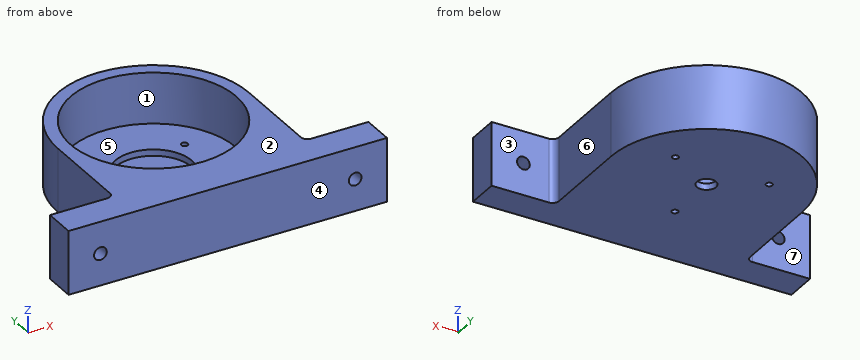
```python
from build123d import *

# Parameters (mm, degrees)
PAD_DEPTH       = 10
SKETCH001_R     = 13
POCKET_DEPTH    = 8
SKETCH002_R     = 6
POCKET001_DEPTH = 1
SKETCH003_R     = 1.5
POCKET002_DEPTH = 1
SKETCH004_R     = 0.5
POCKET003_DEPTH = 2
SKETCH005_R     = 1
POCKET004_DEPTH = 5
FILLET_R        = 1
FILLET001_R     = 1


with BuildPart() as part:
    # Sketch → Pad (new body)
    with BuildSketch(Plane.XY):
        with BuildLine():
            ThreePointArc((15, 0), (0, 15), (-15, 0))
            Line((-15, 0), (-15, -15))
            Line((-15, -15), (-25, -15))
            Line((-25, -15), (-25, -20))
            Line((-25, -20), (25, -20))
            Line((25, -15), (25, -20))
            Line((15, -15), (25, -15))
            Line((15, 0), (15, -15))
        make_face()
    extrude(amount=PAD_DEPTH)

    # Sketch001 (on Face10 of Pad) → Pocket (cut)
    with BuildSketch(Plane.XY.offset(10)):
        Circle(SKETCH001_R)
    extrude(amount=-POCKET_DEPTH, mode=Mode.SUBTRACT)

    # Sketch002 (on Face12 of Pocket) → Pocket001 (cut)
    with BuildSketch(Plane.XY.offset(2)):
        Circle(SKETCH002_R)
    extrude(amount=-POCKET001_DEPTH, mode=Mode.SUBTRACT)

    # Sketch003 (on Face14 of Pocket001) → Pocket002 (cut)
    with BuildSketch(Plane.XY.offset(1)):
        Circle(SKETCH003_R)
    extrude(amount=-POCKET002_DEPTH, mode=Mode.SUBTRACT)

    # Sketch004 (on Face14 of Pocket002) → Pocket003 (cut)
    with BuildSketch(Plane.XY.offset(2)):
        with Locations((0, -8.5)):
            Circle(SKETCH004_R)
        with Locations((7.361216, 4.25)):
            Circle(SKETCH004_R)
        with Locations((-7.361216, 4.25)):
            Circle(SKETCH004_R)
    extrude(amount=-POCKET003_DEPTH, mode=Mode.SUBTRACT)

    # Sketch005 (on Face6 of Pocket003) → Pocket004 (cut)
    with BuildSketch(Plane(origin=(0, -15, 0), x_dir=(-1, 0, 0), z_dir=(0, 1, 0))):
        with Locations((-20, 5)):
            Circle(SKETCH005_R)
        with Locations((20, 5)):
            Circle(SKETCH005_R)
    extrude(amount=-POCKET004_DEPTH, mode=Mode.SUBTRACT)

    # Fillet
    fillet_edges = [part.edges().sort_by_distance(p)[0] for p in [
        (-15, -15, 5),
    ]]
    fillet(fillet_edges, radius=FILLET_R)

    # Fillet001
    fillet001_edges = [part.edges().sort_by_distance(p)[0] for p in [
        (15, -15, 5),
    ]]
    fillet(fillet001_edges, radius=FILLET001_R)


solid = part.part
```
The model under review builds one solid part; all positions refer to its coordinate system, in mm. Face numbers are marked on the shaded views. A direction names the side the tool comes from. Round coordinates to 2 decimals unless told otherwise and drop trailing zeros. Loops run counter-clockwise (first coordinate to the right, second up) from the corner with the lowest first, then second, coordinate; pieces in that order, holes last. Notation, with made-up numbers: M 86.5,32.25 L 112.5,32.25 A30 cw 112.5,65.25 Z; hole C 9,-25.5 d9. An arc over 180 degrees is marked long. Write item = value, one per line.
Item 1: Take a section at C-C on y = -8.5. Write out the cut boundary in (x, z).
Return value:
outline = M -15,0 L -0.5,0 L -0.5,2 L -9.84,2 L -9.84,10 L -15,10 Z; M 0.5,0 L 15,0 L 15,10 L 9.84,10 L 9.84,2 L 0.5,2 Z
Item 2: Take a section at D-D on x = 0. Write out the cut boundary in (y, z).
Return value:
outline = M -20,0 L -9,0 L -9,2 L -13,2 L -13,10 L -20,10 Z; M -8,0 L -1.5,0 L -1.5,1 L -6,1 L -6,2 L -8,2 Z; M 1.5,0 L 15,0 L 15,10 L 13,10 L 13,2 L 6,2 L 6,1 L 1.5,1 Z
Item 3: Take a section at B-B on z = 2.5. Write out the cut boundary in (x, y).
Return value:
outline = M -25,-20 L 25,-20 L 25,-15 L 16,-15 A1 cw 15,-14 L 15,0 A15 ccw -15,0 L -15,-14 A1 cw -16,-15 L -25,-15 Z; hole C 0,0 d26
Item 4: Take a section at A-A on x = 20. Write out the cut boundary in (y, z), then the cut area to 3 significant figures.
Return value:
outline = M -20,0 L -15,0 L -15,4 L -20,4 Z; M -20,6 L -15,6 L -15,10 L -20,10 Z
area = 40.0 mm2
Item 5: The part is to be moulded in two halves that separate along Y. For the marked faces 1, 2 and 3, say which applies: released by +Y, released by -Y, zero draft, split by the parting line, or undercut.
Return value:
face_1 = undercut
face_2 = zero draft
face_3 = released by +Y
Item 6: For line 1 (Y direction, x = 0, z = 0.5); line 2 (Y direction, x = 0, z = 5.5); line 3 (Y direction, x = 0, z = 1.4), list the stretches that pass through material, from the lowest coordinate up. Write a range as [from, to].
Return value:
line_1 = [-20, -9], [-8, -1.5], [1.5, 15]
line_2 = [-20, -13], [13, 15]
line_3 = [-20, -9], [-8, -6], [6, 15]
Item 7: Insertion check: P1, Ø4, axis at x = 0, y = 0, coming from the -Z side; P2, Ø2.5, axis at x = 20, z = 5, coming from the +Y side; P3, Ø1.2, axis at x = -20, z = 5, coming from the +Y side; P4, Ø3, axis at y = -10.5, z = 3, coming from the -X side. Each pin has a flat end and moves straight along its axis. Give the tip position at first contact, or say it passes through.
Return value:
P1 = 0
P2 = -15
P3 = through
P4 = -15
Item 8: Machinability: for the marked faces 4, 5, 6 and 7, which of the approach directions +Z, -Z, +X, -X, +Y, -Y give a long, thin tool a straight path to every point of the face, cutting with its end or side? Answer none if there is none.
Return value:
face_4 = +Z, -Z, +X, -X, -Y
face_5 = +Z
face_6 = +Z, -Z, +X, +Y
face_7 = +Z, -Z, -X, +Y
